Build history of the part. All positions in model axes, mm. Face numbers are marked on the shaded views. A direction names the side the tool comes from. Coordinates: 2 decimals unless noted, no trailing zeros. Write each loop counter-clockwise with the first axis right and the second up, starting at its lowest first coordinate (ties: lowest second). Pieces come first, ordered by that corner, then holes.
```python
from build123d import *

# Parameters (mm, degrees)
F0_R     = 2.1
F1_DEPTH = 26
F3_DEPTH = 20


with BuildPart() as f1:
    # F0 (on Top) → F1 (new body)
    with BuildSketch(Plane.XY):
        with BuildLine():
            ThreePointArc((-12.5, 5.5), (-18, 0), (-12.5, -5.5))
            Line((-12.5, -5.5), (12.5, -5.5))
            ThreePointArc((12.5, -5.5), (18, 0), (12.5, 5.5))
            Line((12.5, 5.5), (-12.5, 5.5))
        make_face()
        with Locations((-12.5, 0)):
            Circle(F0_R, mode=Mode.SUBTRACT)
        with Locations((12.5, 0)):
            Circle(F0_R, mode=Mode.SUBTRACT)
    extrude(amount=F1_DEPTH)

    # F2 (on face) → F3 (cut)
    with BuildSketch(Plane.XY.offset(26)):
        Polygon((10.1, 5.5), (-10.1, 5.5), (-10.1, 0.5), (-10.460392, 0.5), (-10.460392, -0.5), (-10.1, -0.5), (-10.1, -5.5), (10.1, -5.5), (10.1, -0.5), (10.460392, -0.5), (10.460392, 0.5), (10.1, 0.5), align=None)
    extrude(amount=-F3_DEPTH, mode=Mode.SUBTRACT)


solid = f1.part
```
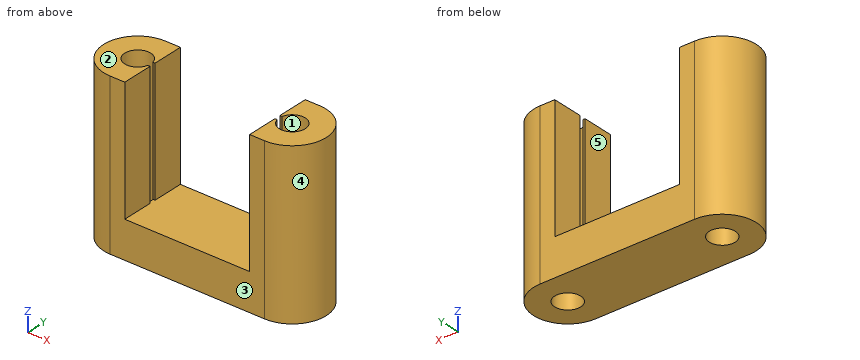
1. Saw through at B-B on z = 23.75. List the corners of the cut face in (x, y).
Computed values:
outline: (-12.5, -5.5) - (-10.1, -5.5) - (-10.1, -0.5) - (-10.46, -0.5) arc R2.1 cw (long way) to (-10.46, 0.5) - (-10.1, 0.5) - (-10.1, 5.5) - (-12.5, 5.5) arc R5.5 ccw to start; (10.1, -5.5) - (12.5, -5.5) arc R5.5 ccw to (12.5, 5.5) - (10.1, 5.5) - (10.1, 0.5) - (10.46, 0.5) arc R2.1 cw (long way) to (10.46, -0.5) - (10.1, -0.5) - close
2. Mould opens along Y. For the marked faces 1, 2 and 3 say: +Y half, -Y half, draft (parallel to the pull), parting line (faces both ways), or undercut.
Computed values:
face 1: undercut
face 2: draft
face 3: -Y half
3. Saw through at D-D on y = 2.5. List the corners of the cut face in (x, z).
Computed values:
outline: (-17.4, 0) - (17.4, 0) - (17.4, 26) - (10.1, 26) - (10.1, 6) - (-10.1, 6) - (-10.1, 26) - (-17.4, 26) - close
4. Saw through at C-C on x = -13. List the corners of the cut face in (y, z), plus the area to 3 significant figures.
Computed values:
outline: (-5.48, 0) - (-2.04, 0) - (-2.04, 26) - (-5.48, 26) - close; (2.04, 0) - (5.48, 0) - (5.48, 26) - (2.04, 26) - close
area: 179 mm2
5. Probe line 1 along X through (y, z) = (0, 5.5); line 2 along Y through (x, z) = (12.5, 10); line 3 along X through (y, z) = (0, 6.25). List the from-to ranges inside material, lowest first.
Computed values:
line 1: x = -18 to -14.6, -10.4 to 10.4, 14.6 to 18
line 2: y = -5.5 to -2.1, 2.1 to 5.5
line 3: x = -18 to -14.6, 14.6 to 18
6. Saw through at A-A on z = 4.5. List the corners of the cut face in (x, y).
Computed values:
outline: (-12.5, -5.5) - (12.5, -5.5) arc R5.5 ccw to (12.5, 5.5) - (-12.5, 5.5) arc R5.5 ccw to start; hole circle Ø4.2 at (-12.5, 0); hole circle Ø4.2 at (12.5, 0)
7. 3-axis set-ups, long thin cutter, end or side, ignore diameter. For the marked faces 4 and 5: which of +Z, -Z, +X, -X, +Y, -Y reach the whole face in a straight line?
Computed values:
face 4: +Z, -Z, +X
face 5: +Z, +Y, -Y
8. Flat gauge pins, fed straight in: pin 1 (3 mm diameter, centred on y = -1, z = 19.5, fed in from +X); pin 2 (4 mm diameter, centred on x = 6.5, z = 15, fed in from +Y); pin 3 (1.5 mm diameter, centred on y = -3.5, z = 18.5, fed in from +X); pin 4 (1 mm diameter, centred on x = 0.5, y = -3, fed in from +Z). Where does each tip first touch, or does it go through?
Computed values:
pin 1: stops at x = 18
pin 2: passes through
pin 3: stops at x = 17.26
pin 4: stops at z = 6
